Can you work these out from the model? Positions are in its coordinate system, mm. A direction names the side the tool comes from. Give positions to 0.01 mm unless a question says otherwise; leave off trailing zeros. One line per item, written item: value.
from build123d import *

# Parameters (mm, degrees)
SKETCH_1_R      = 3
EXTRUDE_1_DEPTH = 450


with BuildPart() as part:
    # 草图1 → 凸台-拉伸1 (new body)
    with BuildSketch(Plane(origin=(0, 0, 0), x_dir=(1, 0, 0), z_dir=(0, 1, 0))):
        with BuildLine():
            Line((-33.25, 15), (-45, 15))
            Line((-45, 15), (-45, 3.25))
            Line((-45, 3.25), (-43.1, 3.25))
            Line((-43.1, 3.25), (-43.1, 5.3))
            Line((-43.1, 5.3), (-36.746672245, 5.3))
            ThreePointArc((-36.746672245, 5.3), (-34.1, 0), (-36.746672245, -5.3))
            Line((-36.746672245, -5.3), (-43.1, -5.3))
            Line((-43.1, -5.3), (-43.1, -3.25))
            Line((-43.1, -3.25), (-45, -3.25))
            Line((-45, -3.25), (-45, -15))
            Line((-45, -15), (-33.25, -15))
            Line((-33.25, -15), (-33.25, -13.1))
            Line((-33.25, -13.1), (-35.3, -13.1))
            Line((-35.3, -13.1), (-35.3, -6.746672245))
            ThreePointArc((-35.3, -6.746672245), (-30, -4.1), (-24.7, -6.746672245))
            Line((-24.7, -6.746672245), (-24.7, -13.1))
            Line((-24.7, -13.1), (-26.75, -13.1))
            Line((-26.75, -13.1), (-26.75, -15))
            Line((-26.75, -15), (-3.25, -15))
            Line((-3.25, -15), (-3.25, -13.1))
            Line((-3.25, -13.1), (-5.3, -13.1))
            Line((-5.3, -13.1), (-5.3, -6.746672245))
            ThreePointArc((-5.3, -6.746672245), (0, -4.1), (5.3, -6.746672245))
            Line((5.3, -6.746672245), (5.3, -13.1))
            Line((5.3, -13.1), (3.25, -13.1))
            Line((3.25, -13.1), (3.25, -15))
            Line((3.25, -15), (26.75, -15))
            Line((26.75, -15), (26.75, -13.1))
            Line((26.75, -13.1), (24.7, -13.1))
            Line((24.7, -13.1), (24.7, -6.746672245))
            ThreePointArc((24.7, -6.746672245), (30, -4.1), (35.3, -6.746672245))
            Line((35.3, -6.746672245), (35.3, -13.1))
            Line((35.3, -13.1), (33.25, -13.1))
            Line((33.25, -13.1), (33.25, -15))
            Line((33.25, -15), (45, -15))
            Line((45, -15), (45, -3.25))
            Line((45, -3.25), (43.1, -3.25))
            Line((43.1, -3.25), (43.1, -5.3))
            Line((43.1, -5.3), (36.746672245, -5.3))
            ThreePointArc((36.746672245, -5.3), (34.1, 0), (36.746672245, 5.3))
            Line((36.746672245, 5.3), (43.1, 5.3))
            Line((43.1, 5.3), (43.1, 3.25))
            Line((43.1, 3.25), (45, 3.25))
            Line((45, 3.25), (45, 15))
            Line((45, 15), (33.25, 15))
            Line((33.25, 15), (33.25, 13.1))
            Line((33.25, 13.1), (35.3, 13.1))
            Line((35.3, 13.1), (35.3, 6.746672245))
            ThreePointArc((35.3, 6.746672245), (30, 4.1), (24.7, 6.746672245))
            Line((24.7, 6.746672245), (24.7, 13.1))
            Line((24.7, 13.1), (26.75, 13.1))
            Line((26.75, 13.1), (26.75, 15))
            Line((26.75, 15), (3.25, 15))
            Line((3.25, 15), (3.25, 13.1))
            Line((3.25, 13.1), (5.3, 13.1))
            Line((5.3, 13.1), (5.3, 6.746672245))
            ThreePointArc((5.3, 6.746672245), (0, 4.1), (-5.3, 6.746672245))
            Line((-5.3, 6.746672245), (-5.3, 13.1))
            Line((-5.3, 13.1), (-3.25, 13.1))
            Line((-3.25, 13.1), (-3.25, 15))
            Line((-3.25, 15), (-26.75, 15))
            Line((-26.75, 15), (-26.75, 13.1))
            Line((-26.75, 13.1), (-24.7, 13.1))
            Line((-24.7, 13.1), (-24.7, 6.746672245))
            ThreePointArc((-24.7, 6.746672245), (-30, 4.1), (-35.3, 6.746672245))
            Line((-35.3, 6.746672245), (-35.3, 13.1))
            Line((-35.3, 13.1), (-33.25, 13.1))
            Line((-33.25, 13.1), (-33.25, 15))
        make_face()
        with Locations(Location((-40, -10, 0), (0, 0, 270))):
            Circle(SKETCH_1_R, mode=Mode.SUBTRACT)
        with Locations(Location((-30, 0, 0), (0, 0, 270))):
            Circle(SKETCH_1_R, mode=Mode.SUBTRACT)
        with Locations(Location((0, 0, 0), (0, 0, 270))):
            Circle(SKETCH_1_R, mode=Mode.SUBTRACT)
        with Locations(Location((40, -10, 0), (0, 0, 270))):
            Circle(SKETCH_1_R, mode=Mode.SUBTRACT)
        with Locations(Location((-40, 10, 0), (0, 0, 270))):
            Circle(SKETCH_1_R, mode=Mode.SUBTRACT)
        with Locations(Location((30, 0, 0), (0, 0, 270))):
            Circle(SKETCH_1_R, mode=Mode.SUBTRACT)
        with Locations(Location((40, 10, 0), (0, 0, 270))):
            Circle(SKETCH_1_R, mode=Mode.SUBTRACT)
    extrude(amount=EXTRUDE_1_DEPTH)


solid = part.part
1) We'd pull the mould along Z, two halves only. Please class faces 1 (the face through (-15, 222, -15)), 2 (the face through (-39, 222, 15)), 3 (the face through (34.1, 221.8, 0.1)): released by +Z, released by -Z, zero draft, split by the parting line, or undercut.
Answer list:
face 1: released by -Z
face 2: released by +Z
face 3: undercut
2) If we section it at A-A (y = 299): State how many separate pieces and enclosed holes the cut face has, and give its area (3 significant figures).
Answer list:
separate pieces: 1
enclosed holes: 7
area: 1,710 mm^2
3) For faces 4 (the face through (30.1, 221.8, -4.1)), 5 (the face through (-15, 222, 15)), which set-ups out of +Z, -Z, +X, -X, +Y, -Y let a thin tool reach every point of the face, with its end or its side?
Answer list:
face 4: +Y, -Y
face 5: +Z, +X, -X, +Y, -Y
4) I need wall thicknesses on L1, parallel to X at y = 20, z = 14.25; L2, parallel to X at y = 155, z = -10; L3, parallel to X at y = 293.5, z = -5. Which ranges of each line are inside material? Lowest first, please.
Answer list:
L1: x = -45 to -33.25, -26.75 to -3.25, 3.25 to 26.75, 33.25 to 45
L2: x = -45 to -43, -37 to -35.3, -24.7 to -5.3, 5.3 to 24.7, 35.3 to 37, 43 to 45
L3: x = -45 to -43.1, -36.38 to -33.34, -26.66 to -3.34, 3.34 to 26.66, 33.34 to 36.38, 43.1 to 45
5) Will this pin go through, and if not, where does the flat tip stop? pin 1 (5.5 mm diameter, centred on x = 40, z = -10, fed in from -Y).
Answer list:
pin 1: passes through
